Drawing for the job (mm, zero at the part's lowest x, y, z). A direction names the side the tool comes from. Round coordinates to 2 decimals unless told otherwise and drop trailing zeros. Write each loop counter-clockwise with the first axis right and the second up, starting at its lowest first coordinate (ties: lowest second). Pieces come first, ordered by that corner, then holes. Notation, with made-up numbers: (70, -3.5) - (113, -3.5) arc R22 cw to (113, 21.5) - close; hole circle Ø5 at (64, 53). An arc over 180 degrees is marked (long way). One line per question, with ' | ' between items.
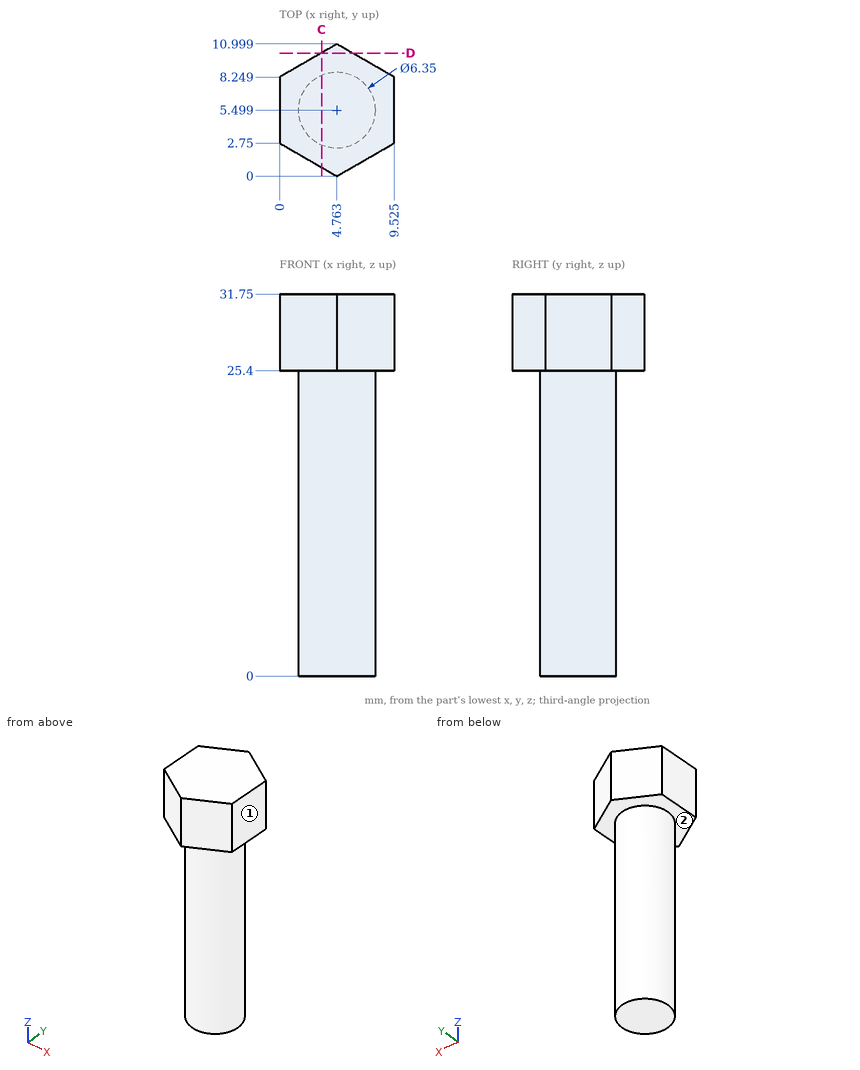
Q1. Saw through at D-D, the plane y = 10.25. List the corners of the cut face in (x, z).
Found:
outline: (3.47, 25.4) - (6.06, 25.4) - (6.06, 31.75) - (3.47, 31.75) - close
Q2. Drop flat-ended pins along their axis: pin 1 (4 mm diameter, centred on y = 3.5, z = 10, fed in from +X); pin 2 (4 mm diameter, centred on x = 2, y = 4.5, fed in from -Z); pin 3 (4 mm diameter, centred on x = 6, z = 22.5, fed in from -Y); pin 4 (1.5 mm diameter, centred on x = 6, z = 27, fed in from -Y). Give the stop position or say it passes through.
Found:
pin 1: x = 7.94 | pin 2: z = 0 | pin 3: y = 2.32 | pin 4: y = 0.28
Q3. Which spindle directions (+Z, -Z, +X, -X, +Y, -Y) get a long thin tool onto all of the face, cutting with end or side? Do the marked faces 1 and 2. Say none if no direction does.
Found:
face 1: +Z, -Z, +X, +Y, -Y | face 2: -Z
Q4. Saw through at C-C, the plane x = 3.5. List the corners of the cut face in (y, z).
Found:
outline: (0.73, 25.4) - (2.59, 25.4) - (2.59, 0) - (8.41, 0) - (8.41, 25.4) - (10.27, 25.4) - (10.27, 31.75) - (0.73, 31.75) - close
Q5. Drill centre lines: L1, parallel to Z at x = 6.75, y = 1.75; L2, parallel to X at y = 5.5, z = 10; L3, parallel to Y at x = 4.75, z = 10 (1 decimal). Where is each one in solid material? Low to high. Write a range as from..to.
Found:
L1: 25.4..31.75 | L2: 1.59..7.94 | L3: 2.3..8.7
